```python
from build123d import *

# Parameters (mm, degrees)
SKETCH_1_R          = 1.5
EXTRUDE_1_DEPTH     = 5
SKETCH_2_R          = 4.9
CUT_EXTRUDE_1_DEPTH = 3.5
CHAMFER_1_SIZE      = 0.3


with BuildPart() as part:
    # ｽｹｯﾁ1 → ﾎﾞｽ - 押し出し1 (new body)
    with BuildSketch(Plane(origin=(0, 0, 0), x_dir=(1, 0, 0), z_dir=(0, 1, 0))):
        with BuildLine():
            Line((-2.557342371, -5.15), (2.557342371, -5.15))
            ThreePointArc((2.557342371, -5.15), (5.75, 0), (2.557342371, 5.15))
            Line((2.557342371, 5.15), (-2.557342371, 5.15))
            ThreePointArc((-2.557342371, 5.15), (-5.75, 0), (-2.557342371, -5.15))
        make_face()
        with Locations(Location((0, 0, 0), (0, 0, 270))):
            Circle(SKETCH_1_R, mode=Mode.SUBTRACT)
    extrude(amount=EXTRUDE_1_DEPTH)

    # ｽｹｯﾁ2 → ｶｯﾄ - 押し出し1 (cut)
    with BuildSketch(Plane.XZ):
        with Locations(Location((0, 0, 0), (0, 0, 270))):
            Circle(SKETCH_2_R)
    extrude(amount=-CUT_EXTRUDE_1_DEPTH, mode=Mode.SUBTRACT)

    # 面取り1
    chamfer_1_edges = [part.edges().sort_by_distance(p)[0] for p in [
        (5.75, 5, 0),
        (-5.75, 5, 0),
        (5.75, 0, 0),
        (-5.75, 0, 0),
    ]]
    chamfer(chamfer_1_edges, length=CHAMFER_1_SIZE)


solid = part.part
```
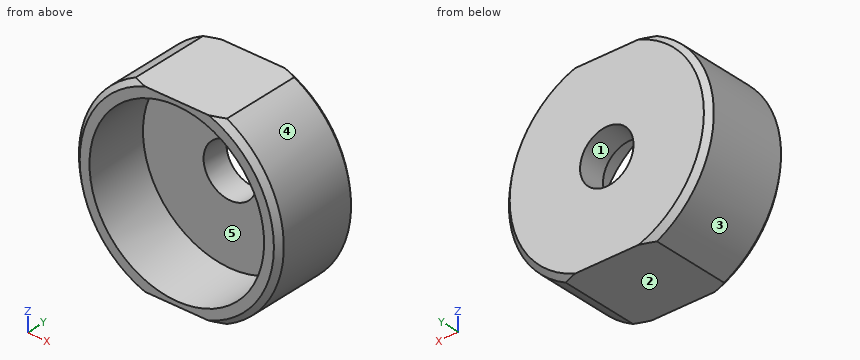
Check sheet for the modelled part. Datum: model origin and axes. Units: mm. Face numbers are marked on the shaded views. A direction names the side the tool comes from. Give positions to 0.01 mm unless a question says otherwise; leave off trailing zeros. Order: outer loops, then holes, each group sorted by start corner. A loop starts at its lowest first (then second) coordinate and runs counter-clockwise, first axis right, second up. Notation, with made-up numbers: (51, -28) -> (108, -28) arc R23 cw to (108, 2) -> close; hole circle Ø2 at (87.5, 80.5). An arc over 180 degrees is marked (long way). Use CSV: the item, a comma, the result in double quotes. Start each with the question number.
1) Sectioned sample at D-D, the plane y = 4.1. Record the boundary of the cut face in (x, z).
2) Sectioned sample at A-A, the plane x = 0. Record the boundary of the cut face in (y, z).
3) Set-up check for the marked faces 4 and 5: record each of +Z, -Z, +X, -X, +Y, -Y from which the full face is reachable in a straight line by a thin tool's end or side.
4) Go/stop test with flat-tipped pins: P1, Ø5, axis at x = 1, z = -1, coming from the -Y side; P2, Ø1.8, axis at x = 0, z = 0, coming from the -Y side. Record where each tip stops, or that it passes through.
5) Sectioned sample at B-B, the plane z = 0. Record the boundary of the cut face in (x, y).
6) Sectioned sample at C-C, the plane y = 1.3. Record the boundary of the cut face in (x, z).
7) Mould release check, pull along Z, two halves, no side actions. Record for the marked faces 1, 2 and 3: released by +Z, released by -Z, zero draft, split by the parting line, or undercut.
8) Material ranges on line 1 (Z direction, x = 0, y = 4.35); line 2 (Y direction, x = 1.75, z = 1); line 3 (Z direction, x = 1.25, y = 4.5), recorded low to high. Write a range as from..to.
Recorded:
1,outline,"(-2.56, -5.15) -> (2.56, -5.15) arc R5.75 ccw to (2.56, 5.15) -> (-2.56, 5.15) arc R5.75 ccw to start; hole circle Ø3 at (0, 0)"
2,outline,"(0, -5.15) -> (5, -5.15) -> (5, -1.5) -> (3.5, -1.5) -> (3.5, -4.9) -> (0, -4.9) -> close; (0, 4.9) -> (3.5, 4.9) -> (3.5, 1.5) -> (5, 1.5) -> (5, 5.15) -> (0, 5.15) -> close"
3,face 4,"+X, +Y, -Y"
3,face 5,"-Y"
4,P1,"y = 3.5"
4,P2,"through"
5,outline,"(-5.75, 0.3) -> (-5.45, 0) -> (-4.9, 0) -> (-4.9, 3.5) -> (-1.5, 3.5) -> (-1.5, 5) -> (-5.45, 5) -> (-5.75, 4.7) -> close; (1.5, 3.5) -> (4.9, 3.5) -> (4.9, 0) -> (5.45, 0) -> (5.75, 0.3) -> (5.75, 4.7) -> (5.45, 5) -> (1.5, 5) -> close"
6,outline,"(-2.56, -5.15) -> (2.56, -5.15) arc R5.75 ccw to (2.56, 5.15) -> (-2.56, 5.15) arc R5.75 ccw to start; hole circle Ø9.8 at (0, 0)"
7,face 1,"undercut"
7,face 2,"released by -Z"
7,face 3,"split by the parting line"
8,line 1,"-5.15..-1.5, 1.5..5.15"
8,line 2,"3.5..5"
8,line 3,"-5.15..-0.83, 0.83..5.15"
